Part model, mm, in its own coordinate system. Face numbers are marked on the shaded views. A direction names the side the tool comes from. Give positions to 0.01 mm unless a question says otherwise; leave off trailing zeros. Write each loop counter-clockwise with the first axis right and the second up, starting at its lowest first coordinate (ties: lowest second). Pieces come first, ordered by that corner, then holes. Notation, with made-up numbers: M 19,86 L 45,86 A21 cw 45,95 Z; hole C 20,40 d2. An arc over 180 degrees is marked long. Use a Markdown table: item, result.
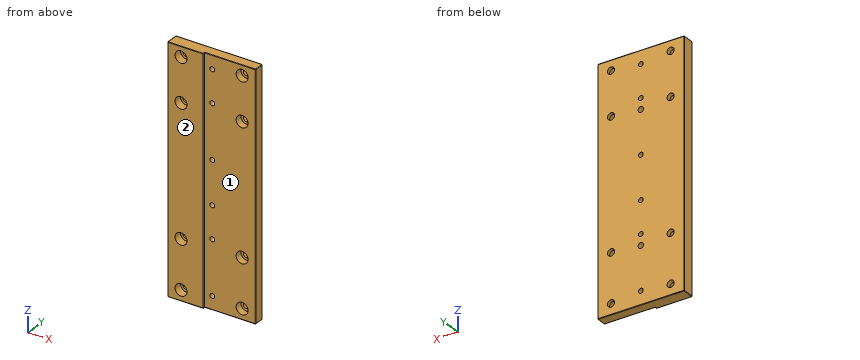
```python
from build123d import *

# Parameters (mm, degrees)
F0_W           = 66
F0_H           = 450
F1_DEPTH       = 23
F0_W_2         = 94
F2_DEPTH       = 19
F3_D           = 10
F3_DEPTH       = 12
F3_TIP         = 3.0043030951
F4_D           = 8.8
F4_DEPTH       = 33
F4_TIP         = 2.6437867237
F6_D           = 13
F6_DEPTH       = 30
F6_CBORE_D     = 22
F6_CBORE_DEPTH = 15
F6_TIP         = 3.9055940237
F8_D           = 13
F8_DEPTH       = 30
F8_CBORE_D     = 22
F8_CBORE_DEPTH = 13
F8_TIP         = 3.9055940237
F9_R           = 1


with BuildPart() as f1:
    # F0 (on Front) → F1 (new body)
    with BuildSketch(Plane.XZ):
        with Locations((-47, 0)):
            Rectangle(F0_W, F0_H)
    extrude(amount=F1_DEPTH)

    # F0 (on Front) → F2 (join)
    with BuildSketch(Plane.XZ):
        with Locations((33, 0)):
            Rectangle(F0_W_2, F0_H)
    extrude(amount=F2_DEPTH)

    # F3
    with Locations(Plane(origin=(0, 0, 0), x_dir=(1, 0, 0), z_dir=(0, 1, 0))):
        with Locations((0, 120), (0, -120)):
            Hole(F3_D / 2, depth=F3_DEPTH)
            with Locations((0, 0, -(F3_DEPTH + F3_TIP / 2))):  # 118° drill point
                Cone(0, F3_D / 2, F3_TIP, mode=Mode.SUBTRACT)

    # F4
    with Locations(Plane(origin=(0, 0, 0), x_dir=(1, 0, 0), z_dir=(0, 1, 0))):
        with Locations((0, 200), (0, 100), (0, 40), (0, -40), (0, -140), (0, -200)):
            Hole(F4_D / 2, depth=F4_DEPTH)
            with Locations((0, 0, -(F4_DEPTH + F4_TIP / 2))):  # 118° drill point
                Cone(0, F4_D / 2, F4_TIP, mode=Mode.SUBTRACT)

    # F6
    with Locations(Plane.XZ.offset(23)):
        with Locations((-55, 206), (-55, 125), (-55, -115), (-55, -205)):
            CounterBoreHole(F6_D / 2, F6_CBORE_D / 2, F6_CBORE_DEPTH, depth=F6_DEPTH)
            with Locations((0, 0, -(F6_DEPTH + F6_TIP / 2))):  # 118° drill point
                Cone(0, F6_D / 2, F6_TIP, mode=Mode.SUBTRACT)

    # F8
    with Locations(Plane.XZ.offset(19)):
        with Locations((55, 206), (55, 125), (55, -115), (55, -205)):
            CounterBoreHole(F8_D / 2, F8_CBORE_D / 2, F8_CBORE_DEPTH, depth=F8_DEPTH)
            with Locations((0, 0, -(F8_DEPTH + F8_TIP / 2))):  # 118° drill point
                Cone(0, F8_D / 2, F8_TIP, mode=Mode.SUBTRACT)

    # F9
    f9_edges = [f1.edges().sort_by_distance(p)[0] for p in [
        (-80, -11.5, 225),
        (-80, -11.5, -225),
        (-80, 0, 0),
        (-80, -23, 0),
        (-14, -21, 225),
        (-47, -23, 225),
        (0, 0, 225),
        (80, -9.5, 225),
        (33, -19, 225),
        (80, -9.5, -225),
        (80, 0, 0),
        (80, -19, 0),
        (-47, -23, -225),
        (-14, -21, -225),
        (33, -19, -225),
        (0, 0, -225),
    ]]
    fillet(f9_edges, radius=F9_R)


solid = f1.part
```
1. Drop flat-ended pins along their axis: P1, Ø11.5, axis at x = 0, z = -100, coming from the -Y side; P2, Ø10.5, axis at x = 55, z = 206, coming from the +Y side; P3, Ø1, axis at y = -20.5, z = 137.5, coming from the +X side; P4, Ø15, axis at x = 55, z = 125, coming from the -Y side. Give the stop position or say it passes through.
Findings below:
| item | result |
|---|---|
| P1 | y = -19 |
| P2 | through |
| P3 | x = -14 |
| P4 | y = -6 |
2. Cut at D-D, the plane x = -56.5. State how many separate pieces and enclosed holes the cut face has, then the cut area to 3 significant figures.
Findings below:
| item | result |
|---|---|
| separate pieces | 5 |
| enclosed holes | 0 |
| area | 8,640 mm2 |
3. Drill centre lines: L1, parallel to Z at x = -55, y = -3; L2, parallel to Y at x = 26, z = -28; L3, parallel to X at y = -20, z = -17. Where is each one in solid material? Low to high.
Findings below:
| item | result |
|---|---|
| L1 | -225 to -211.5, -198.5 to -121.5, -108.5 to 118.5, 131.5 to 199.5, 212.5 to 225 |
| L2 | -19 to 0 |
| L3 | -80 to -14 |
4. Cut at C-C, the plane z = -138. Give the cut face in (x, y).
Findings below:
| item | result |
|---|---|
| outline | M -80,-22 A1 ccw -79,-23 L -14,-23 L -14,-19 L 79,-19 A1 ccw 80,-18 L 80,-1 A1 ccw 79,0 L -79,0 A1 ccw -80,-1 Z |
5. Cut at B-B, the plane x = 70.5. Give the cut face in (y, z).
Findings below:
| item | result |
|---|---|
| outline | M -19,-224 A1 ccw -18,-225 L -1,-225 A1 ccw 0,-224 L 0,224 A1 ccw -1,225 L -18,225 A1 ccw -19,224 Z |
6. Cut at A-A, the plane z = 140. Give the cut face in (x, y).
Findings below:
| item | result |
|---|---|
| outline | M -80,-22 A1 ccw -79,-23 L -14,-23 L -14,-19 L -4.4,-19 L -4.4,0 L -79,0 A1 ccw -80,-1 Z; M 4.4,-19 L 79,-19 A1 ccw 80,-18 L 80,-1 A1 ccw 79,0 L 4.4,0 Z |
7. Tool access for the marked faces 1 and 2: list every direction of +Z, -Z, +X, -X, +Y, -Y with a clear straight run to the whole face (end or side of a thin tool).
Findings below:
| item | result |
|---|---|
| face 1 | +Z, -Z, +X, -Y |
| face 2 | +Z, -Z, +X, -X, -Y |
